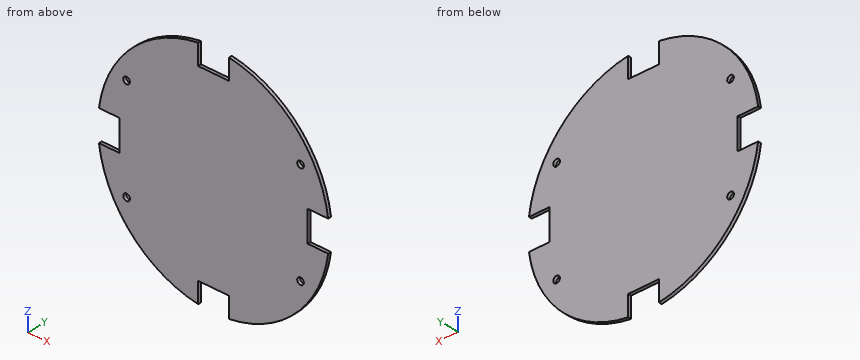
from build123d import *

# Parameters (mm, degrees)
SKETCH1_R           = 1.651
BOSS_EXTRUDE1_DEPTH = 1.5875


with BuildPart() as part:
    # Sketch1 → Boss-Extrude1 (new body)
    with BuildSketch(Plane(origin=(0, 0, 0), x_dir=(1, 0, 0), z_dir=(0, 1, 0))):
        with BuildLine():
            Line((-7.62, 56.896), (-7.62, 46.736))
            Line((-7.62, 46.736), (7.62, 46.736))
            Line((7.62, 46.736), (7.62, 56.896))
            ThreePointArc((7.62, 56.896), (40.590757667, 40.590757667), (56.896, 7.62))
            Line((56.896, 7.62), (46.736, 7.62))
            Line((46.736, 7.62), (46.736, -7.62))
            Line((46.736, -7.62), (56.896, -7.62))
            ThreePointArc((56.896, -7.62), (40.590757667, -40.590757667), (7.62, -56.896))
            Line((7.62, -56.896), (7.62, -46.736))
            Line((7.62, -46.736), (-7.62, -46.736))
            Line((-7.62, -46.736), (-7.62, -56.896))
            ThreePointArc((-7.62, -56.896), (-40.590757667, -40.590757667), (-56.896, -7.62))
            Line((-56.896, -7.62), (-46.736, -7.62))
            Line((-46.736, -7.62), (-46.736, 7.62))
            Line((-46.736, 7.62), (-56.896, 7.62))
            ThreePointArc((-56.896, 7.62), (-40.590757667, 40.590757667), (-7.62, 56.896))
        make_face()
        with Locations(Location((-43.18, 25.4, 0), (0, 0, 270))):
            Circle(SKETCH1_R, mode=Mode.SUBTRACT)
        with Locations(Location((-43.18, -25.4, 0), (0, 0, 270))):
            Circle(SKETCH1_R, mode=Mode.SUBTRACT)
        with Locations(Location((43.18, -25.4, 0), (0, 0, 270))):
            Circle(SKETCH1_R, mode=Mode.SUBTRACT)
        with Locations(Location((43.18, 25.4, 0), (0, 0, 270))):
            Circle(SKETCH1_R, mode=Mode.SUBTRACT)
    extrude(amount=BOSS_EXTRUDE1_DEPTH)


solid = part.part
Model file for the job. Use its own axes, mm. Give positions to 0.01 mm unless a question says otherwise; leave off trailing zeros. Write each loop counter-clockwise with the first axis right and the second up, starting at its lowest first coordinate (ties: lowest second). Pieces come first, ordered by that corner, then holes. Notation, with made-up numbers: (-30, 40.5) - (-10, 40.5) arc R20 ccw to (-10, 70.5) - close; hole circle Ø11 at (42.25, 37). An arc over 180 degrees is marked (long way). Answer as CSV lines item,"result".
1. Band-saw the part on D-D (z = 25.4). Write the cut outline in (x, y).
Responses:
outline,"(-51.48, 0) - (-44.83, 0) - (-44.83, 1.59) - (-51.48, 1.59) - close; (-41.53, 0) - (41.53, 0) - (41.53, 1.59) - (-41.53, 1.59) - close; (44.83, 0) - (51.48, 0) - (51.48, 1.59) - (44.83, 1.59) - close"
2. Drill centre lines: L1, parallel to X at y = 0.85, z = -25.4; L2, parallel to Z at x = 4.5, y = 0.45. Where is each one in solid material? Low to high. Write a range as [from, to].
Responses:
L1,"x = [-51.48, -44.83], [-41.53, 41.53], [44.83, 51.48]"
L2,"z = [-46.74, 46.74]"
3. Band-saw the part on C-C (x = -49). Write the cut outline in (y, z).
Responses:
outline,"(0, -29.9) - (1.59, -29.9) - (1.59, -7.62) - (0, -7.62) - close; (0, 7.62) - (1.59, 7.62) - (1.59, 29.9) - (0, 29.9) - close"
4. Band-saw the part on B-B (z = 48.5). Write the cut outline in (x, y).
Responses:
outline,"(-30.71, 0) - (-7.62, 0) - (-7.62, 1.59) - (-30.71, 1.59) - close; (7.62, 0) - (30.71, 0) - (30.71, 1.59) - (7.62, 1.59) - close"
5. Pin check, flat tips, straight feed: pin 1 (4 mm diameter, centred on x = -44, z = -3.5, fed in from -Y); pin 2 (2.5 mm diameter, centred on x = -43.18, z = -25.4, fed in from -Y); pin 3 (0.8 mm diameter, centred on x = 51, y = 1, fed in from +Z); pin 4 (0.8 mm diameter, centred on x = -49.5, y = 0.5, fed in from +Z). Stop position of each tip, or through.
Responses:
pin 1,"stops at y = 0"
pin 2,"passes through"
pin 3,"stops at z = 27.11"
pin 4,"stops at z = 29.74"
6. Band-saw the part on A-A (y = 1.15). Write the cut outline in (x, z).
Responses:
outline,"(-56.9, -7.62) arc R57.4 ccw to (-7.62, -56.9) - (-7.62, -46.74) - (7.62, -46.74) - (7.62, -56.9) arc R57.4 ccw to (56.9, -7.62) - (46.74, -7.62) - (46.74, 7.62) - (56.9, 7.62) arc R57.4 ccw to (7.62, 56.9) - (7.62, 46.74) - (-7.62, 46.74) - (-7.62, 56.9) arc R57.4 ccw to (-56.9, 7.62) - (-46.74, 7.62) - (-46.74, -7.62) - close; hole circle Ø3.3 at (-43.18, -25.4); hole circle Ø3.3 at (-43.18, 25.4); hole circle Ø3.3 at (43.18, -25.4); hole circle Ø3.3 at (43.18, 25.4)"
